Read the model definition and answer for the solid it produces. Units are mm, in the model's axes. A direction names the side the tool comes from. Coordinates: 2 decimals unless noted, no trailing zeros. Loops run counter-clockwise (first coordinate to the right, second up) from the corner with the lowest first, then second, coordinate; pieces in that order, holes last. Notation, with made-up numbers: (26, -20) -> (69, -20) arc R15 ccw to (69, -14) -> close; hole circle Ø1 at (64.25, 81.25). An arc over 180 degrees is marked (long way). Answer as a JSON object with one key per item and string values. Group by question number.
1) Section B-B, the plane y = 10 is taken. Give the vertices of the cut face in (x, z), plus the area to 3 significant figures.
2) Section D-D, the plane x = 33 is taken. Give the vertices of the cut face in (y, z).
3) A flat-ended cylindrical pin translates along its axis: P1, Ø6.5, axis at x = 16, y = 13.5, coming from the +Z side. Find the tip coordinate at first contact, or state that the pin passes through.
4) Determine the mould class of faces 4 (the face through (38.1, 13, 16)), 5 (the face through (20, 13, 6.35)), 6 (the face through (28.531, 13, 3)), 7 (the face through (19, 22, 31.75)) for opening direction X: released by +X, released by -X, zero draft, split by the parting line, or undercut.
5) Section C-C, the plane z = 27.5 is taken. Give the vertices of the cut face in (x, y), plus the area to 3 significant figures.
6) Section A-A, the plane z = 5.5 is taken. Give the vertices of the cut face in (x, y).
7) Consider probe 1 along X at (y, z) = (12.75, 3.5); probe 2 along Y at (x, z) = (32, 26.5); probe 3 along Z at (x, y) = (16, 4.25). Determine where each line is inside the solid, lowest interval first. Write a range as [from, to].
8) Which of the six approach directions +Z, -Z, +X, -X, +Y, -Y give full straight-line access (tool end or side, diameter ignored) to faces 1 (the face through (19, 19.523, 29)), 2 (the face through (10.854, 13, 3)), 3 (the face through (19, 3, 31.75))?
from build123d import *

# Parameters (mm, degrees)
F0_W     = 25.4
F0_H     = 31.75
F1_DEPTH = 38.1
F2_W     = 38.1
F2_H     = 12.7
F3_DEPTH = 6.35
F4_W     = 17.676627
F4_H     = 25.4
F5_DEPTH = 6.35


with BuildPart() as f1:
    # F0 (on Right) → F1 (new body)
    with BuildSketch(Plane.YZ):
        with Locations((12.7, 15.875)):
            Rectangle(F0_W, F0_H)
    extrude(amount=F1_DEPTH)

    # F2 (on face) → F3 (cut)
    with BuildSketch(Plane.XY.offset(31.75)):
        with Locations((19.05, 13.172559)):
            Rectangle(F2_W, F2_H)
    extrude(amount=-F3_DEPTH, mode=Mode.SUBTRACT)

    # F4 (on face) → F5 (cut)
    with BuildSketch(Plane(origin=(0, 0, 0), x_dir=(1, 0, 0), z_dir=(0, 0, -1))):
        with Locations((19.692383, -12.7)):
            Rectangle(F4_W, F4_H)
    extrude(amount=-F5_DEPTH, mode=Mode.SUBTRACT)


solid = f1.part
Determined:
{
 "1": {"outline": "(0, 0) -> (10.85, 0) -> (10.85, 6.35) -> (28.53, 6.35) -> (28.53, 0) -> (38.1, 0) -> (38.1, 25.4) -> (0, 25.4) -> close", "area": "855 mm²"},
 "2": {"outline": "(0, 0) -> (25.4, 0) -> (25.4, 31.75) -> (19.52, 31.75) -> (19.52, 25.4) -> (6.82, 25.4) -> (6.82, 31.75) -> (0, 31.75) -> close"},
 "3": {"P1": "z = 25.4"},
 "4": {"face 4": "released by +X", "face 5": "undercut", "face 6": "undercut", "face 7": "zero draft"},
 "5": {"outline": "(0, 0) -> (38.1, 0) -> (38.1, 6.82) -> (0, 6.82) -> close; (0, 19.52) -> (38.1, 19.52) -> (38.1, 25.4) -> (0, 25.4) -> close", "area": "484 mm²"},
 "6": {"outline": "(0, 0) -> (10.85, 0) -> (10.85, 25.4) -> (0, 25.4) -> close; (28.53, 0) -> (38.1, 0) -> (38.1, 25.4) -> (28.53, 25.4) -> close"},
 "7": {"probe 1": "[0, 10.85], [28.53, 38.1]", "probe 2": "[0, 6.82], [19.52, 25.4]", "probe 3": "[6.35, 31.75]"},
 "8": {"face 1": "+Z, +X, -X", "face 2": "-Z, +Y, -Y", "face 3": "+Z, +X, -X, +Y, -Y"}
}
